```python
from build123d import *

# Parameters (mm, degrees)
BOSS_EXTRUDE1_DEPTH = 24
BOSS_EXTRUDE2_DEPTH = 28
SKETCH1_4_W         = 71
SKETCH1_4_H         = 11
BOSS_EXTRUDE3_DEPTH = 71
SKETCH1_5_W         = 71
SKETCH1_5_H         = 13
BOSS_EXTRUDE4_DEPTH = 54
SKETCH2_W           = 26
SKETCH2_H           = 8
CUT_EXTRUDE1_DEPTH  = 96
CHAMFER1_SIZE       = 20


with BuildPart() as part:
    # Sketch1 → Boss-Extrude1 (new body)
    with BuildSketch(Plane(origin=(0, 0, 0), x_dir=(1, 0, 0), z_dir=(0, 1, 0))):
        Polygon((0, 47), (0, 0), (95, 0), (95, 82), (71, 82), (71, 71), (71, 58), (71, 47), align=None)
        with BuildLine():
            ThreePointArc((25, 14.5), (13.5, 26), (25, 37.5))
            Line((25, 37.5), (70, 37.5))
            ThreePointArc((70, 37.5), (81.5, 26), (70, 14.5))
            Line((70, 14.5), (25, 14.5))
        make_face(mode=Mode.SUBTRACT)
    extrude(amount=BOSS_EXTRUDE1_DEPTH)

    # Sketch1_3 → Boss-Extrude2 (add)
    with BuildSketch(Plane(origin=(0, 0, 0), x_dir=(1, 0, 0), z_dir=(0, 1, 0))):
        with BuildLine():
            Line((25, 14.5), (70, 14.5))
            ThreePointArc((70, 14.5), (81.5, 26), (70, 37.5))
            Line((70, 37.5), (25, 37.5))
            ThreePointArc((25, 37.5), (13.5, 26), (25, 14.5))
        make_face()
        with BuildLine():
            ThreePointArc((25, 32.5), (18.5, 26), (25, 19.5))
            Line((25, 19.5), (70, 19.5))
            ThreePointArc((70, 19.5), (76.5, 26), (70, 32.5))
            Line((70, 32.5), (25, 32.5))
        make_face(mode=Mode.SUBTRACT)
    extrude(amount=BOSS_EXTRUDE2_DEPTH)

    # Sketch1_4 → Boss-Extrude3 (add)
    with BuildSketch(Plane(origin=(0, 0, 0), x_dir=(1, 0, 0), z_dir=(0, 1, 0))):
        with Locations((35.5, 76.5)):
            Rectangle(SKETCH1_4_W, SKETCH1_4_H)
        with Locations((35.5, 52.5)):
            Rectangle(SKETCH1_4_W, SKETCH1_4_H)
    extrude(amount=BOSS_EXTRUDE3_DEPTH)

    # Sketch1_5 → Boss-Extrude4 (add)
    with BuildSketch(Plane(origin=(0, 0, 0), x_dir=(1, 0, 0), z_dir=(0, 1, 0))):
        with Locations((35.5, 64.5)):
            Rectangle(SKETCH1_5_W, SKETCH1_5_H)
    extrude(amount=BOSS_EXTRUDE4_DEPTH)

    # Sketch2 → Cut-Extrude1 (cut)
    with BuildSketch(Plane(origin=(95, 0, 0), x_dir=(0, 0, -1), z_dir=(1, 0, 0))):
        with Locations((26, 4)):
            Rectangle(SKETCH2_W, SKETCH2_H)
    extrude(amount=-CUT_EXTRUDE1_DEPTH, mode=Mode.SUBTRACT)

    # Chamfer1
    chamfer1_edges = [part.edges().sort_by_distance(p)[0] for p in [
        (71, 71, -76.5),
    ]]
    chamfer(chamfer1_edges, length=CHAMFER1_SIZE)


solid = part.part
```
Part model, mm, in its own coordinate system. A direction names the side the tool comes from. Round coordinates to 2 decimals unless told otherwise and drop trailing zeros. Loops run counter-clockwise (first coordinate to the right, second up) from the corner with the lowest first, then second, coordinate; pieces in that order, holes last. Notation, with made-up numbers: (56, 32.5) -> (70, 32.5) arc R20 cw to (70, 59.5) -> close; hole circle Ø6 at (-7, 11.25). An arc over 180 degrees is marked (long way). Use CSV: the item, a comma, the result in double quotes. Start each with the question number.
1) Which spindle directions (+Z, -Z, +X, -X, +Y, -Y) get a long thin tool onto all of the face, cutting with end or side? Do faces 4 (the flat face through (34, 54, -65)), 5 (the cylindrical face through (81.497, 25.972, -25.747)), 6 (the flat face through (47, 18, -19.5)). Say none if no direction does.
2) Drop flat-ended pins along their axis: P1, Ø1.2, axis at x = 52, y = 25.5, coming from the +Z side; P2, Ø23.5, axis at x = 21.5, y = 50, coming from the +Z side; P3, Ø22, axis at x = 56.5, y = 16.5, coming from the +Z side; P4, Ø4, axis at x = 82.5, z = -17.5, coming from the +Y side. Give the stop position or say it passes through.
3) Wall check: L1, parallel to Z at x = 35, y = 27; L2, parallel to Z at x = 87, y = 4; L3, parallel to Z at x = 27, y = 66. Give the ranges that are in metal, low to high. Write a range as [from, to].
4) Cut at C-C, the plane z = -26. Write the cut outline in (x, y).
5) Cut at B-B, the plane x = 59.5. Write the cut outline in (y, z), plus the area to 3 significant figures.
6) Cut at A-A, the plane y = 66. Write the cut outline in (x, z).
7) Pull direction Z, two halves, no side cores. Call faces 1 (the flat face through (47, 12, 0)), 2 (the flat face through (48, 26, -37.5)), 3 (the flat face through (25, 71, -53)): +Z half, -Z half, draft (parallel to the pull), parting line (faces both ways), or undercut.
8) Cut at D-D, the plane y = 18.5. Write the cut outline in (x, z), plus the area to 3 significant figures.
Determined:
1,face 4,"+X, -X, +Y"
1,face 5,"+X, +Y"
1,face 6,"+Y, -Y"
2,P1,"stops at z = -14.5"
2,P2,"stops at z = -47"
2,P3,"stops at z = 0"
2,P4,"stops at y = 24"
3,L1,"z = [-82, -47], [-37.5, -32.5], [-19.5, -14.5]"
3,L2,"z = [-82, -39], [-13, 0]"
3,L3,"z = [-82, -71], [-58, -47]"
4,outline,"(0, 8) -> (18.5, 8) -> (18.5, 28) -> (13.5, 28) -> (13.5, 24) -> (0, 24) -> close; (76.5, 8) -> (95, 8) -> (95, 24) -> (81.5, 24) -> (81.5, 28) -> (76.5, 28) -> close"
5,outline,"(0, -82) -> (62.5, -82) -> (62.5, -71) -> (54, -71) -> (54, -58) -> (62.5, -58) -> (62.5, -47) -> (24, -47) -> (24, -37.5) -> (28, -37.5) -> (28, -32.5) -> (8, -32.5) -> (8, -39) -> (0, -39) -> close; (0, -13) -> (8, -13) -> (8, -19.5) -> (28, -19.5) -> (28, -14.5) -> (24, -14.5) -> (24, 0) -> (0, 0) -> close"
5,area,"2,830 mm2"
6,outline,"(0, -82) -> (56, -82) -> (56, -71) -> (0, -71) -> close; (0, -58) -> (56, -58) -> (56, -47) -> (0, -47) -> close"
7,face 1,"+Z half"
7,face 2,"undercut"
7,face 3,"draft"
8,outline,"(0, -82) -> (95, -82) -> (95, 0) -> (0, 0) -> close; hole (25, -32.5) -> (70, -32.5) arc R6.5 ccw to (70, -19.5) -> (25, -19.5) arc R6.5 ccw to start"
8,area,"7,070 mm2"
